The model under review builds one solid part; all positions refer to its coordinate system, in mm. Give positions to 0.01 mm unless a question says otherwise; leave off trailing zeros. Order: outer loops, then holes, each group sorted by start corner. A loop starts at its lowest first (then second) coordinate and runs counter-clockwise, first axis right, second up. Notation, with made-up numbers: (71, 15.25) -> (87, 15.25) arc R29 cw to (87, 36.25) -> close; hole circle Ø3 at (49, 37.25). An arc over 180 degrees is marked (long way). Use one line per item in the form item = value.
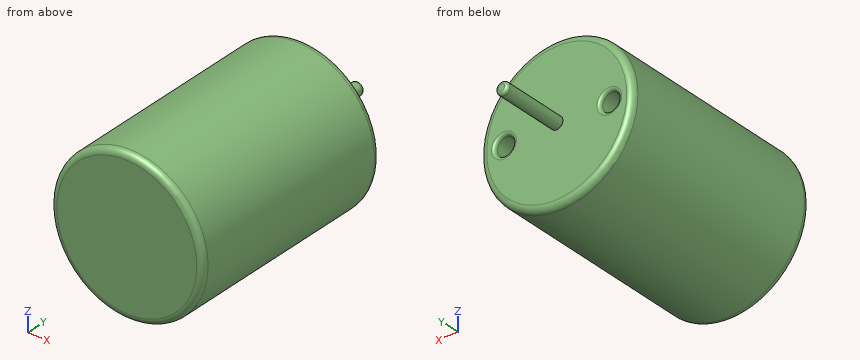
Autodesk Inventor part; units mm, degrees
ref_plane "YZ Plane" through (0, 0, 0) normal (1, 0, 0) x (0, 1, 0)
ref_plane "XZ Plane" through (0, 0, 0) normal (0, 1, 0) x (-1, 0, 0)
ref_plane "XY Plane" through (0, 0, 0) normal (0, 0, 1) x (1, 0, 0)
sketch "Sketch2" plane through (0, 0, 0) normal (0, 1, 0) x (-1, 0, 0)
  circle A0 centre (0, 0) radius 12.3
  dimension "d1" = 24.6
extrude "Extrusion1" add sketch "Sketch2" along normal blind 35.2
sketch "Sketch3" plane through (0, 35.2, 0) normal (0, 1, 0) x (1, 0, 0)
  circle A0 centre (0, 0) radius 1
  dimension "d4" = 2
extrude "Extrusion2" add sketch "Sketch3" along normal blind 11
sketch "Sketch4" plane through (0, 35.2, 0) normal (0, 1, 0) x (1, 0, 0)
  circle A0 centre (-8.5, 0) radius 1.5
  circle A1 centre (8.5, 0) radius 1.5
  point P0 (0, 0)
  dimension "d7" = 3
  dimension "d9" = 8.5
  dimension "d13" = 360
extrude "Extrusion3" cut sketch "Sketch4" against normal blind 17
fillet "Fillet1" radius 1 2 edges at (12.3, 35.2, 0) (12.3, 0, 0)
fillet "Fillet1" radius 0.5 3 edges at (7, 35.2, 0) (-1, 46.2, 0) (-10, 35.2, 0)
properties part number "RS-385 Dc Electric Motor"
1. For L1, parallel to Y at x = 9.25, z = -5.25; L2, parallel to Z at x = 8.5, y = 27; L3, parallel to X at y = 10.5, z = -1, list the stretches that pass through material, from the lowest coordinate up.
Values:
L1 = 0 to 35.2
L2 = -8.89 to -1.5, 1.5 to 8.89
L3 = -12.26 to 12.26
2. Add section A-A on y = 20. Give the boundary of the cut face in (x, z).
Values:
outline = circle Ø24.6 at (0, 0); hole circle Ø3 at (-8.5, 0); hole circle Ø3 at (8.5, 0)
3. For pin 1 Ø5 at (y, z) = (23, 8.5) entering from +X; pin 2 Ø1.5 at (x, z) = (4.5, 6.5) entering from +Y; pin 3 Ø2.5 at (x, z) = (8.5, 0) entering from +Y, all flat-tipped, find the tip position at first contact; note any pin that passes through.
Values:
pin_1 = 10.74
pin_2 = 35.2
pin_3 = 18.2
